```python
from build123d import *

# Parameters (mm, degrees)
F0_W     = 200
F0_H     = 200
F1_DEPTH = 25
F3_DEPTH = 25
F4_W     = 43.039545
F4_H     = 37.170328
F5_DEPTH = 4.644


with BuildPart() as f1:
    # F0 (on Front) → F1 (new body)
    with BuildSketch(Plane.XZ):
        with Locations((-100, -100)):
            Rectangle(F0_W, F0_H)
    extrude(amount=F1_DEPTH)

    # F2 (on face) → F3 (join)
    with BuildSketch(Plane.XZ.offset(25)):
        with BuildLine():
            ThreePointArc((-149.452707, -53.410247), (-147.62081, -50.344453), (-146.983063, -46.830449))
            ThreePointArc((-146.983063, -46.830449), (-166.345315, -43.316446), (-149.452707, -53.410247))
        make_face()
        with BuildLine():
            ThreePointArc((-23.562095, -110.983481), (-62.478073, -54.809964), (-128.744229, -71.504692))
            ThreePointArc((-128.744229, -71.504692), (-104.646117, -167.156998), (-23.562095, -110.983481))
        make_face()
    extrude(amount=F3_DEPTH)

    # F4 (on face) → F5 (join)
    with BuildSketch(Plane.XZ.offset(25)):
        with Locations((-164.246566, -39.92312)):
            Rectangle(F4_W, F4_H)
    extrude(amount=F5_DEPTH)


solid = f1.part
```
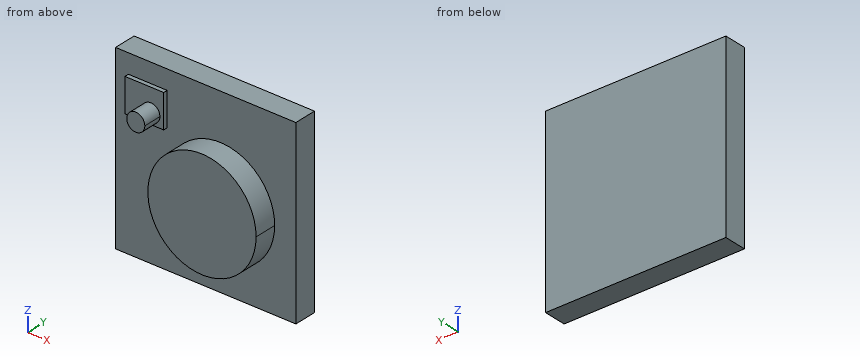
Part model, mm, in its own coordinate system. Give positions to 0.01 mm unless a question says otherwise; leave off trailing zeros. Loops run counter-clockwise (first coordinate to the right, second up) from the corner with the lowest first, then second, coordinate; pieces in that order, holes last. Notation, with made-up numbers: M 37.5,-4.5 L 45.5,-4.5 A21 cw 45.5,8.5 Z; hole C -24,59 d8. An arc over 180 degrees is marked long. Return JSON: item names as keys, results as strings.
1) Drill centre lines: line 1 (Y direction, x = -173.5, z = -165); line 2 (Z direction, x = -72, y = -48); line 3 (X direction, y = -27.5, z = -42.5). Where is each one in solid material? Low to high.
Calculated:
{"line 1": "y = -25 to 0", "line 2": "z = -169.86 to -52.11", "line 3": "x = -185.77 to -142.73"}
2) Saw through at C-C, the plane z = -120.5. List the corners of the cut face in (x, y).
Calculated:
{"outline": "M -200,-25 L -142.8,-25 L -142.8,-50 L -24.32,-50 L -24.32,-25 L 0,-25 L 0,0 L -200,0 Z"}
3) Saw through at D-D, the plane x = -88. List the corners of the cut face in (y, z), then the cut area to 3 significant figures.
Calculated:
{"outline": "M -50,-170.82 L -25,-170.82 L -25,-200 L 0,-200 L 0,0 L -25,0 L -25,-51.15 L -50,-51.15 Z", "area": "7,990 mm2"}
4) Saw through at A-A, the plane y = -32.5. List the corners of the cut face in (x, z).
Calculated:
{"outline": "M -149.45,-53.41 A10 ccw -146.98,-46.83 A10 ccw long Z; C -83.56,-110.98 d120"}
5) Saw through at B-B, the plane x = -162.5. List the corners of the cut face in (y, z), then the cut area to 3 significant figures.
Calculated:
{"outline": "M -50,-55.17 L -29.64,-55.17 L -29.64,-58.51 L -25,-58.51 L -25,-200 L 0,-200 L 0,0 L -25,0 L -25,-21.34 L -29.64,-21.34 L -29.64,-38.49 L -50,-38.49 Z", "area": "5,510 mm2"}
6) Flat gauge pins, fed straight in: pin 1 Ø3 at (x, y) = (-78.5, -31) entering from -Z; pin 2 Ø1.4 at (y, z) = (-28.5, -46) entering from -X; pin 3 Ø5 at (x, z) = (-163.5, -64.5) entering from -Y. Where does each tip first touch, or does it go through?
Calculated:
{"pin 1": "stops at z = -170.88", "pin 2": "stops at x = -185.77", "pin 3": "stops at y = -25"}
